```python
from build123d import *

# Parameters (mm, degrees)
SKETCH1_W           = 200
SKETCH1_H           = 200
BOSS_EXTRUDE1_DEPTH = 10
SKETCH2_W           = 20
SKETCH2_H           = 20
CUT_EXTRUDE2_DEPTH  = 3
SKETCH3_W           = 20
SKETCH3_H           = 15
SKETCH3_W_2         = 15
SKETCH3_H_2         = 20
CUT_EXTRUDE3_DEPTH  = 3


with BuildPart() as part:
    # Sketch1 → Boss-Extrude1 (new body)
    with BuildSketch(Plane.XY):
        with Locations((-100, -100)):
            Rectangle(SKETCH1_W, SKETCH1_H)
    extrude(amount=BOSS_EXTRUDE1_DEPTH)

    # Sketch2 → Cut-Extrude2 (cut)
    with BuildSketch(Plane.XY.offset(10)):
        with Locations((-100, -100)):
            Rectangle(SKETCH2_W, SKETCH2_H)
    extrude(amount=-CUT_EXTRUDE2_DEPTH, mode=Mode.SUBTRACT)

    # Sketch3 → Cut-Extrude3 (cut)
    with BuildSketch(Plane.XY.offset(10)):
        with Locations((-100, -47.5)):
            Rectangle(SKETCH3_W, SKETCH3_H)
        with Locations((-47.5, -100)):
            Rectangle(SKETCH3_W_2, SKETCH3_H_2)
    extrude(amount=-CUT_EXTRUDE3_DEPTH, mode=Mode.SUBTRACT)


solid = part.part
```
For this review, take the finished solid that the model builds, in its own axes (mm). A direction names the side the tool comes from. Round coordinates to 2 decimals unless told otherwise and drop trailing zeros. Loops run counter-clockwise (first coordinate to the right, second up) from the corner with the lowest first, then second, coordinate; pieces in that order, holes last.
(1) Mouldability with a two-part tool opening along Y and no side actions: class faces 3 (the flat face through (-101, -121, 10)), 4 (the flat face through (-101, 0, 5)), 5 (the flat face through (-100, -100, 7)), 6 (the flat face through (-100, -47, 7)) as released by +Y, released by -Y, zero draft, split by the parting line, or undercut.
Returned:
face 3: zero draft
face 4: released by +Y
face 5: undercut
face 6: undercut
(2) Clearance check with flat-ended pins moving along their axes: P1, Ø1, axis at x = -113, y = -154.5, coming from the -Z side; P2, Ø6, axis at x = -104.5, y = -100, coming from the +Z side. State where each tip first meets the part, or that it passes through.
Returned:
P1: stops at z = 0
P2: stops at z = 7
(3) Wall thickness on line 1 along Y through (x, z) = (-40.5, 7.5): over which ranges is the line inside the solid? List them lowest first.
Returned:
line 1: y = -200 to -110, -90 to 0
(4) We need section B-B (y = -101). Give the boundary of the cut face in (x, z).
Returned:
outline: (-200, 0) - (0, 0) - (0, 10) - (-40, 10) - (-40, 7) - (-55, 7) - (-55, 10) - (-90, 10) - (-90, 7) - (-110, 7) - (-110, 10) - (-200, 10) - close
(5) We need section A-A (y = -46.5). Give the boundary of the cut face in (x, z), plus the area to 3 significant figures.
Returned:
outline: (-200, 0) - (0, 0) - (0, 10) - (-90, 10) - (-90, 7) - (-110, 7) - (-110, 10) - (-200, 10) - close
area: 1,940 mm2
(6) Tool access review of faces 1 (the flat face through (-48, -100, 7)), 2 (the flat face through (-101, -200, 5)): name each direction out of +Z, -Z, +X, -X, +Y, -Y from which nothing blocks a thin tool from reaching the whole face with its end or side.
Returned:
face 1: +Z
face 2: +Z, -Z, +X, -X, -Y
